```python
from build123d import *

# Parameters (mm, degrees)
SKETCH2_R           = 7.9375
SKETCH2_R_2         = 3.2639
BOSS_EXTRUDE1_DEPTH = 19.05
SKETCH3_W           = 15.555026682
SKETCH3_H           = 25.4
CUT_EXTRUDE1_DEPTH  = 12.7
SKETCH4_R           = 3.2639
CUT_EXTRUDE2_DEPTH  = 28.240315825


with BuildPart() as part:
    # Sketch2 → Boss-Extrude1 (new body)
    # profile 1 of 2: a face of its own
    with BuildSketch(Plane(origin=(0, 0, 0), x_dir=(0, 0, -1), z_dir=(1, 0, 0))):
        with BuildLine():
            ThreePointArc((7.9375, 0), (0, -7.9375), (-7.9375, 0))
            Line((-7.9375, 0), (-7.9375, -17.78))
            Line((-7.9375, -17.78), (7.9375, -17.78))
            Line((7.9375, -17.78), (7.9375, 0))
        make_face()
    # profile 2 of 2: a face of its own
    with BuildSketch(Plane(origin=(0, 0, 0), x_dir=(0, 0, -1), z_dir=(1, 0, 0))):
        Circle(SKETCH2_R)
        with Locations(Location((0, 0, 0), (0, 0, 180))):
            Circle(SKETCH2_R_2, mode=Mode.SUBTRACT)
    extrude(amount=BOSS_EXTRUDE1_DEPTH)

    # Sketch3 → Cut-Extrude1 (cut, symmetric)
    with BuildSketch(Plane.XY):
        with Locations((9.494486659, -3.302)):
            Rectangle(SKETCH3_W, SKETCH3_H)
    extrude(amount=CUT_EXTRUDE1_DEPTH, both=True, mode=Mode.SUBTRACT)

    # Sketch4 → Cut-Extrude2 (cut, through all)
    with BuildSketch(Plane(origin=(0, 0, 0), x_dir=(1, 0, 0), z_dir=(0, 1, 0))):
        with Locations(Location((9.525, -0.0635, 0), (0, 0, 270))):
            Circle(SKETCH4_R)
    extrude(amount=-CUT_EXTRUDE2_DEPTH, mode=Mode.SUBTRACT)


solid = part.part
```
Geometry: final body of the model. Coordinates: model frame, mm. A direction names the side the tool comes from. Coordinates: 2 decimals unless noted, no trailing zeros. Order: outer loops, then holes, each group sorted by start corner. A loop starts at its lowest first (then second) coordinate and runs counter-clockwise, first axis right, second up. Notation, with made-up numbers: M -2.5,68 L 47.5,68 A15 ccw 47.5,86 Z; hole C 44,38.25 d11. An arc over 180 degrees is marked long. Answer in a Markdown table with one row per item. Add a question column.
Q1. Reachability of faces 4 (the flat face through (13, -16.002, 0)), 5 (the flat face through (0, -5, 0)) from +Z, -Z, +X, -X, +Y, -Y: full face, straight path, thin tool, end or side. Return the list, or none.
Q2. Section query D-D on x = 16.25. Return the cut outline in (y, z), and give its area (3 significant figures).
Q3. Section query A-A on y = -8. Return the cut outline in (x, z).
Q4. Section query B-B on z = 0. Return the cut outline in (x, y).
Q5. Contact query for a flat-ended pin moving along its axis: P1, Ø3, axis at y = -6, z = 3.5, coming from the -X side. Output: stop coordinate, or through.
Q6. Line query: L1, parallel to X at y = 2, z = 4; L2, parallel to Y at x = 1.1, z = 0; L3, parallel to Y at x = 2.25, z = -6.5. Output: solid intervals per line, ascending.
Q7. Mould query, pull axis Y, two halves, no side actions, for faces 1 (the flat face through (1.717, -4, 0)), 2 (the cylindrical face through (18.149, 3.186, -0.708)), 3 (the cylindrical face through (0.846, 7.936, -0.175)). Classes: released by +Y, released by -Y, zero draft, split by the parting line, or undercut.
Q8. Section query C-C on y = -0.5. Return the cut outline in (x, z), and give its area (3 significant figures).
Completed:
| question | item | result |
|---|---|---|
| 1 | face 4 | +Z, -Z, +Y |
| 1 | face 5 | +Z, -Z, -X, +Y, -Y |
| 2 | outline | M -17.78,-7.94 L -16,-7.94 L -16,7.94 L -17.78,7.94 Z |
| 2 | area | 28.2 mm2 |
| 3 | outline | M 0,-7.94 L 1.72,-7.94 L 1.72,7.94 L 0,7.94 Z; M 17.27,-7.94 L 19.05,-7.94 L 19.05,7.94 L 17.27,7.94 Z |
| 4 | outline | M 0,-17.78 L 6.26,-17.78 L 6.26,-16 L 1.72,-16 L 1.72,-3.26 L 0,-3.26 Z; M 0,3.26 L 1.72,3.26 L 1.72,7.94 L 0,7.94 Z; M 12.79,-17.78 L 19.05,-17.78 L 19.05,-3.26 L 17.27,-3.26 L 17.27,-16 L 12.79,-16 Z; M 17.27,3.26 L 19.05,3.26 L 19.05,7.94 L 17.27,7.94 Z |
| 5 | P1 | stops at x = 0 |
| 6 | L1 | x = 0 to 1.72, 17.27 to 19.05 |
| 6 | L2 | y = -17.78 to -3.26, 3.26 to 7.94 |
| 6 | L3 | y = -17.78 to -16 |
| 7 | face 1 | zero draft |
| 7 | face 2 | undercut |
| 7 | face 3 | released by +Y |
| 8 | outline | M 0,-7.94 L 1.72,-7.94 L 1.72,-3.23 L 0,-3.23 Z; M 0,3.23 L 1.72,3.23 L 1.72,7.94 L 0,7.94 Z; M 17.27,-7.94 L 19.05,-7.94 L 19.05,-3.23 L 17.27,-3.23 Z; M 17.27,3.23 L 19.05,3.23 L 19.05,7.94 L 17.27,7.94 Z |
| 8 | area | 32.9 mm2 |
